```python
from build123d import *

# Parameters (mm, degrees)
SKETCH1_W           = 50
SKETCH1_H           = 35
SKETCH1_R           = 2.5
BOSS_EXTRUDE1_DEPTH = 6
CUT_EXTRUDE1_DEPTH  = 1
FILLET3_R           = 1


with BuildPart() as part:
    # Sketch1 → Boss-Extrude1 (new body)
    with BuildSketch(Plane.XY):
        Rectangle(SKETCH1_W, SKETCH1_H)
        with Locations((18, 10)):
            Circle(SKETCH1_R, mode=Mode.SUBTRACT)
        with Locations(Location((18, -10, 0), (0, 0, 180))):
            Circle(SKETCH1_R, mode=Mode.SUBTRACT)
        with Locations(Location((-18, 10, 0), (0, 0, 180))):
            Circle(SKETCH1_R, mode=Mode.SUBTRACT)
        with Locations((-18, -10)):
            Circle(SKETCH1_R, mode=Mode.SUBTRACT)
        with BuildLine():
            Line((-7, 4), (7, 4))
            ThreePointArc((7, 4), (7.707106781, 3.707106781), (8, 3))
            Line((8, 3), (8, -3))
            ThreePointArc((8, -3), (7.707106781, -3.707106781), (7, -4))
            Line((7, -4), (-7, -4))
            ThreePointArc((-7, -4), (-7.707106781, -3.707106781), (-8, -3))
            Line((-8, -3), (-8, 3))
            ThreePointArc((-8, 3), (-7.707106781, 3.707106781), (-7, 4))
        make_face(mode=Mode.SUBTRACT)
    extrude(amount=BOSS_EXTRUDE1_DEPTH)

    # Sketch2 → Cut-Extrude1 (cut)
    with BuildSketch(Plane.XY):
        with BuildLine():
            Line((-10.8, -11), (10.8, -11))
            ThreePointArc((10.8, -11), (10.941421356, -10.941421356), (11, -10.8))
            Line((11, -10.8), (11, 10.8))
            ThreePointArc((11, 10.8), (10.941421356, 10.941421356), (10.8, 11))
            Line((10.8, 11), (-10.8, 11))
            ThreePointArc((-10.8, 11), (-10.941421356, 10.941421356), (-11, 10.8))
            Line((-11, 10.8), (-11, -10.8))
            ThreePointArc((-11, -10.8), (-10.941421356, -10.941421356), (-10.8, -11))
        make_face()
        with BuildLine():
            Line((-9.8, -10), (9.8, -10))
            ThreePointArc((9.8, -10), (9.941421356, -9.941421356), (10, -9.8))
            Line((10, -9.8), (10, 9.8))
            ThreePointArc((10, 9.8), (9.941421356, 9.941421356), (9.8, 10))
            Line((9.8, 10), (-9.8, 10))
            ThreePointArc((-9.8, 10), (-9.941421356, 9.941421356), (-10, 9.8))
            Line((-10, 9.8), (-10, -9.8))
            ThreePointArc((-10, -9.8), (-9.941421356, -9.941421356), (-9.8, -10))
        make_face(mode=Mode.SUBTRACT)
    extrude(amount=CUT_EXTRUDE1_DEPTH, mode=Mode.SUBTRACT)

    # Fillet3
    fillet3_edges = [part.edges().sort_by_distance(p)[0] for p in [
        (-7.707106781, 3.707106781, 0),
        (-8, 0, 0),
        (-7.707106781, -3.707106781, 0),
        (0, -4, 0),
        (7.707106781, -3.707106781, 0),
        (8, 0, 0),
        (0, 4, 0),
        (7.707106781, 3.707106781, 0),
    ]]
    fillet(fillet3_edges, radius=FILLET3_R)


solid = part.part
```
Read the model definition and answer for the solid it produces. Units are mm, in the model's axes. A direction names the side the tool comes from. Round coordinates to 2 decimals unless told otherwise and drop trailing zeros. Write each loop counter-clockwise with the first axis right and the second up, starting at its lowest first coordinate (ties: lowest second). Pieces come first, ordered by that corner, then holes. Notation, with made-up numbers: (76.5, 86.25) -> (128.5, 86.25) arc R25 ccw to (128.5, 113.25) -> close; hole circle Ø5 at (66.25, 61.5). An arc over 180 degrees is marked (long way). Answer in a Markdown table with one row per item. Add a question column.
1) Find section D-D, the plane z = 4.55. Determine the outline of the cut face in (x, y).
2) Determine the mould class of faces 4 (the face through (-11, 0.2, 0.5)), 5 (the face through (-8, 0, 3)), 6 (the face through (0, 17.5, 3)), 7 (the face through (25, 0, 3)) for opening direction X: pulls with the +X half, pulls with the -X half, needs draft (parallel to the pull), parting line crosses it, or undercut.
3) Which of the six approach directions +Z, -Z, +X, -X, +Y, -Y give full straight-line access (tool end or side, diameter ignored) to faces 1 (the face through (0, 8, 6)), 2 (the face through (7.715, -3.699, 3.465)), 3 (the face through (0.1, 10, 0.5))?
4) Find section A-A, the plane x = 18. Determine the outline of the cut face in (y, z).
5) Consider line 1 (Y direction, x = 18, z = 2.65); line 2 (Y direction, x = -6, z = 0.85); line 3 (X direction, y = -4.5, z = 0.85). Determine where each line is inside the solid, lowest interval first.
6) Find section C-C, the plane x = 0. Determine the outline of the cut face in (y, z), and give its area (3 significant figures).
7) Given P1, Ø8, axis at x = -18, y = -10, coming from the -Z side, flat-ended and moving along its own axis, determine where the tip first touches the part or whether it passes through.
8) Find section B-B, the plane y = -0.5. Determine the outline of the cut face in (x, z), and give its area (3 significant figures).
Findings below:
| question | item | result |
|---|---|---|
| 1 | outline | (-25, -17.5) -> (25, -17.5) -> (25, 17.5) -> (-25, 17.5) -> close; hole circle Ø5 at (-18, -10); hole circle Ø5 at (-18, 10); hole (-8, -3) arc R1 ccw to (-7, -4) -> (7, -4) arc R1 ccw to (8, -3) -> (8, 3) arc R1 ccw to (7, 4) -> (-7, 4) arc R1 ccw to (-8, 3) -> close; hole circle Ø5 at (18, -10); hole circle Ø5 at (18, 10) |
| 2 | face 4 | undercut |
| 2 | face 5 | undercut |
| 2 | face 6 | needs draft |
| 2 | face 7 | pulls with the +X half |
| 3 | face 1 | +Z, +X, -X, +Y, -Y |
| 3 | face 2 | +Z, -Z |
| 3 | face 3 | -Z |
| 4 | outline | (-17.5, 0) -> (-12.5, 0) -> (-12.5, 6) -> (-17.5, 6) -> close; (-7.5, 0) -> (7.5, 0) -> (7.5, 6) -> (-7.5, 6) -> close; (12.5, 0) -> (17.5, 0) -> (17.5, 6) -> (12.5, 6) -> close |
| 5 | line 1 | -17.5 to -12.5, -7.5 to 7.5, 12.5 to 17.5 |
| 5 | line 2 | -17.5 to -11, -10 to -4.01, 4.01 to 10, 11 to 17.5 |
| 5 | line 3 | -25 to -11, -10 to 10, 11 to 25 |
| 6 | outline | (-17.5, 0) -> (-11, 0) -> (-11, 1) -> (-10, 1) -> (-10, 0) -> (-5, 0) arc R1 ccw to (-4, 1) -> (-4, 6) -> (-17.5, 6) -> close; (4, 1) arc R1 ccw to (5, 0) -> (10, 0) -> (10, 1) -> (11, 1) -> (11, 0) -> (17.5, 0) -> (17.5, 6) -> (4, 6) -> close |
| 6 | area | 160 mm² |
| 7 | P1 | z = 0 |
| 8 | outline | (-25, 0) -> (-11, 0) -> (-11, 1) -> (-10, 1) -> (-10, 0) -> (-9, 0) arc R1 ccw to (-8, 1) -> (-8, 6) -> (-25, 6) -> close; (8, 1) arc R1 ccw to (9, 0) -> (10, 0) -> (10, 1) -> (11, 1) -> (11, 0) -> (25, 0) -> (25, 6) -> (8, 6) -> close |
| 8 | area | 202 mm² |
